```python
from build123d import *

# Parameters (mm, degrees)
SKETCH_1_R          = 1.75
EXTRUDE_1_DEPTH     = 6
SKETCH_2_R          = 3
CUT_EXTRUDE_1_DEPTH = 4


with BuildPart() as part:
    # Эскиз1 → Бобышка-Вытянуть1 (new body)
    with BuildSketch(Plane(origin=(0, 0, 0), x_dir=(1, 0, 0), z_dir=(0, 1, 0))):
        with BuildLine():
            Line((0, 105.25), (12.5, 105.25))
            ThreePointArc((12.5, 105.25), (14.267766953, 105.982233047), (15, 107.75))
            Line((15, 107.75), (15, 108.75))
            ThreePointArc((15, 108.75), (15.732233047, 110.517766953), (17.5, 111.25))
            Line((17.5, 111.25), (118.5, 111.25))
            ThreePointArc((118.5, 111.25), (120.267766953, 110.517766953), (121, 108.75))
            Line((121, 108.75), (121, 107.75))
            ThreePointArc((121, 107.75), (121.732233047, 105.982233047), (123.5, 105.25))
            Line((123.5, 105.25), (136, 105.25))
            ThreePointArc((136, 105.25), (140.471073351, 101.259414462), (137.012279745, 96.365334708))
            Line((137.012279745, 96.365334708), (129.613763077, 94.657252548))
            ThreePointArc((129.613763077, 94.657252548), (124.08407631, 91.197188523), (121.864397453, 85.063469865))
            Line((121.864397453, 85.063469865), (121.379494275, 52.722536916))
            ThreePointArc((121.379494275, 52.722536916), (121.35096588, 52.279643163), (121.278949063, 51.841713576))
            Line((121.278949063, 51.841713576), (109.898949063, -0.948286424))
            ThreePointArc((109.898949063, -0.948286424), (107.58711076, -3.986724053), (103.772892877, -4.155370138))
            Line((103.772892877, -4.155370138), (65.954927395, 11.563007621))
            ThreePointArc((65.954927395, 11.563007621), (61.344389675, 12.298967601), (56.902251647, 10.861572422))
            Line((56.902251647, 10.861572422), (32.846596964, -3.839724299))
            ThreePointArc((32.846596964, -3.839724299), (27.805357329, -3.604011776), (26.153333782, 1.164685703))
            Line((26.153333782, 1.164685703), (36.221084572, 38.73804317))
            ThreePointArc((36.221084572, 38.73804317), (36.853849051, 42.519294597), (36.753491079, 46.35181094))
            Line((36.753491079, 46.35181094), (32.158216583, 83.777318367))
            ThreePointArc((32.158216583, 83.777318367), (29.42615307, 89.505208638), (23.797099717, 92.435508339))
            Line((23.797099717, 92.435508339), (-1.006615848, 96.364030947))
            ThreePointArc((-1.006615848, 96.364030947), (-4.471401388, 101.256527029), (0, 105.25))
        make_face()
        with Locations(Location((35, 105.75, 0), (0, 0, 270))):
            Circle(SKETCH_1_R, mode=Mode.SUBTRACT)
        with Locations(Location((110, 105.75, 0), (0, 0, 270))):
            Circle(SKETCH_1_R, mode=Mode.SUBTRACT)
        with Locations(Location((116.88, 52.79, 0), (0, 0, 270))):
            Circle(SKETCH_1_R, mode=Mode.SUBTRACT)
        with Locations(Location((45.62, 47.74, 0), (0, 0, 270))):
            Circle(SKETCH_1_R, mode=Mode.SUBTRACT)
        with Locations(Location((0, 100.75, 0), (0, 0, 270))):
            Circle(SKETCH_1_R, mode=Mode.SUBTRACT)
        with Locations(Location((136, 100.75, 0), (0, 0, 270))):
            Circle(SKETCH_1_R, mode=Mode.SUBTRACT)
        with Locations(Location((30.5, 0, 0), (0, 0, 270))):
            Circle(SKETCH_1_R, mode=Mode.SUBTRACT)
        with Locations(Location((105.5, 0, 0), (0, 0, 270))):
            Circle(SKETCH_1_R, mode=Mode.SUBTRACT)
        with BuildLine():
            Line((48, 104.25), (103, 104.25))
            ThreePointArc((103, 104.25), (110.123874635, 101.267863648), (112.998876167, 94.100082036))
            Line((112.998876167, 94.100082036), (112.500284745, 60.846202729))
            ThreePointArc((112.500284745, 60.846202729), (111.186497255, 56.039384402), (107.716068497, 52.46340003))
            Line((107.716068497, 52.46340003), (64.817208881, 26.246326643))
            ThreePointArc((64.817208881, 26.246326643), (60.375070853, 24.808931464), (55.764533132, 25.544891444))
            Line((55.764533132, 25.544891444), (51.232831469, 27.428414202))
            ThreePointArc((51.232831469, 27.428414202), (48.311891769, 29.292595834), (46.202504042, 32.041694834))
            ThreePointArc((46.202504042, 32.041694834), (45.33035863, 35.010535959), (45.650081265, 38.088267701))
            ThreePointArc((45.650081265, 38.088267701), (46.871495682, 40.400347733), (48.856177376, 42.102876976))
            ThreePointArc((48.856177376, 42.102876976), (52.06452504, 48.587406051), (47.288889887, 54.02210208))
            ThreePointArc((47.288889887, 54.02210208), (43.80810358, 56.18938194), (42.138332857, 59.934357378))
            Line((42.138332857, 59.934357378), (38.074538484, 93.031306566))
            ThreePointArc((38.074538484, 93.031306566), (40.510442792, 100.876200482), (48, 104.25))
        make_face(mode=Mode.SUBTRACT)
        with BuildLine():
            Line((112.820087132, 41.07481604), (105.561751128, 7.404556143))
            ThreePointArc((105.561751128, 7.404556143), (104.534267438, 6.054139419), (102.83905949, 5.979185604))
            Line((102.83905949, 5.979185604), (74.366820735, 17.81317505))
            ThreePointArc((74.366820735, 17.81317505), (73.140400732, 19.505501844), (74.091491917, 21.366550355))
            Line((74.091491917, 21.366550355), (109.822066675, 43.202820805))
            ThreePointArc((109.822066675, 43.202820805), (112.022629186, 43.127194072), (112.820087132, 41.07481604))
        make_face(mode=Mode.SUBTRACT)
        with BuildLine():
            Line((47.62796861, 15.74134871), (38.316811752, 10.050957756))
            ThreePointArc((38.316811752, 10.050957756), (36.076260803, 10.155718878), (35.342028115, 12.275139979))
            Line((35.342028115, 12.275139979), (37.647028294, 20.87751776))
            ThreePointArc((37.647028294, 20.87751776), (38.695388466, 22.154160251), (40.346483113, 22.206710843))
            Line((40.346483113, 22.206710843), (47.352639792, 19.294724015))
            ThreePointArc((47.352639792, 19.294724015), (48.579059795, 17.602397221), (47.62796861, 15.74134871))
        make_face(mode=Mode.SUBTRACT)
    extrude(amount=EXTRUDE_1_DEPTH)

    # Эскиз2 → Вырез-Вытянуть1 (cut)
    with BuildSketch(Plane(origin=(0, 0, 0), x_dir=(-1, 0, 0), z_dir=(0, -1, 0))):
        with Locations(Location((-110, 105.75, 0), (0, 0, 90))):
            Circle(SKETCH_2_R)
        with Locations(Location((-35, 105.75, 0), (0, 0, 90))):
            Circle(SKETCH_2_R)
        with Locations(Location((-116.88, 52.79, 0), (0, 0, 90))):
            Circle(SKETCH_2_R)
        with Locations(Location((-45.62, 47.74, 0), (0, 0, 90))):
            Circle(SKETCH_2_R)
    extrude(amount=-CUT_EXTRUDE_1_DEPTH, mode=Mode.SUBTRACT)


solid = part.part
```
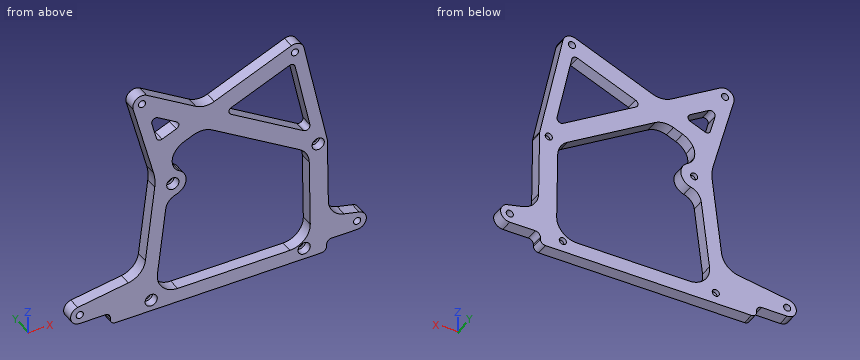
Can you work these out from the model? Positions are in its coordinate system, mm. Give positions to 0.01 mm unless a question says otherwise; leave off trailing zeros. Order: outer loops, then holes, each group sorted by start corner. A loop starts at its lowest first (then second) coordinate and runs counter-clockwise, first axis right, second up. Notation, with made-up numbers: M 61,7.5 L 112,7.5 A12 ccw 112,17.5 Z; hole C 4,55 d9. An arc over 180 degrees is marked long. Write item = value, one per line. Start each with the question number.
Q1. I need wall thicknesses on probe 1 along X at (y, z) = (5.4, -52.79); probe 2 along Z at (x, y) = (99, 1.85); probe 3 along X at (y, z) = (5.3, -47.74). Which ranges of each line are inside material? Lowest first, please. Write a range as [from, to].
Q2. Suppose I cut it at A-A (x = 93). Write out the boundary of the cut face in (y, z), plus the area to 3 significant figures.
Q3. Will these pins go through, and if not, where does the flat tip stop? pin 1 Ø8 at (x, z) = (93, -45.5) entering from +Y; pin 2 Ø3 at (x, y) = (6, 1.5) entering from -Z; pin 3 Ø2 at (x, z) = (0, -100.75) entering from +Y; pin 4 Ø2 at (y, z) = (1.5, -52) entering from -X.
Q4. Suppose I cut it at D-D (y = 1.1). Count the separate pieces of the cut face and the enclosed holes in it, plus the area to 3 significant figures.
Q5. Suppose I cut it at C-C (x = 116.88). Write out the boundary of the cut face in (y, z), plus the area to 3 significant figures.
Q6. Suppose I cut it at B-B (z = -72). Write out the boundary of the cut face in (x, y).
Check result:
q1.probe_1 = [35.96, 49.71], [108.22, 115.13], [118.63, 121.38]
q1.probe_2 = [-111.25, -104.25], [-47.14, -36.59], [-7.57, 2.17]
q1.probe_3 = [36.58, 43.87], [47.37, 52.12], [99.99, 120.39]
q2.outline = M 0,-111.25 L 6,-111.25 L 6,-104.25 L 0,-104.25 Z; M 0,-43.47 L 6,-43.47 L 6,-32.92 L 0,-32.92 Z; M 0,-10.07 L 6,-10.07 L 6,-0.32 L 0,-0.32 Z
q2.area = 164 mm2
q3.pin_1 = 6
q3.pin_2 = -105.25
q3.pin_3 = through
q3.pin_4 = 35.94
q4.separate_pieces = 1
q4.enclosed_holes = 11
q4.area = 4,310 mm2
q5.outline = M 0,-111.25 L 6,-111.25 L 6,-54.54 L 4,-54.54 L 4,-55.79 L 0,-55.79 Z; M 0,-49.79 L 4,-49.79 L 4,-51.04 L 6,-51.04 L 6,-31.44 L 0,-31.44 Z
q5.area = 448 mm2
q6.outline = M 33.6,0 L 40.66,0 L 40.66,6 L 33.6,6 Z; M 112.67,0 L 121.67,0 L 121.67,6 L 112.67,6 Z
